Model file for the job. Use its own axes, mm. A direction names the side the tool comes from. Give positions to 0.01 mm unless a question says otherwise; leave off trailing zeros. Order: outer loops, then holes, each group sorted by start corner. A loop starts at its lowest first (then second) coordinate and runs counter-clockwise, first axis right, second up. Notation, with made-up numbers: (83, 27) - (103, 27) arc R24 cw to (103, 56) - close; hole circle Ø9 at (59.25, 47). An arc over 180 degrees is marked (long way). Return JSON: item names as keys, results as strings. Group by question number.
from build123d import *

# Parameters (mm, degrees)
SKETCH1_W           = 25.4
SKETCH1_H           = 25.4
BOSS_EXTRUDE1_DEPTH = 2.54
BOSS_EXTRUDE3_DEPTH = 2.54
SKETCH6_W           = 25.4
SKETCH6_H           = 3.81
CUT_EXTRUDE1_DEPTH  = 51.545361805
SKETCH7_R           = 1
CUT_EXTRUDE2_DEPTH  = 49.742196298


with BuildPart() as part:
    # Sketch1 → Boss-Extrude1 (new body)
    with BuildSketch(Plane.XY):
        with Locations((12.7, -12.7)):
            Rectangle(SKETCH1_W, SKETCH1_H)
    extrude(amount=BOSS_EXTRUDE1_DEPTH)

    # Sketch2 → Boss-Extrude3 (add, symmetric)
    with BuildSketch(Plane(origin=(0, -19.05, 0), x_dir=(1, 0, 0), z_dir=(0, 1, 0))):
        Polygon((2.286, -35.56), (2.286, -2.54), (12.7, -2.54), (23.114, -2.54), (23.114, -35.56), align=None)
    extrude(amount=BOSS_EXTRUDE3_DEPTH, both=True)

    # Sketch6 → Cut-Extrude1 (cut, through all)
    with BuildSketch(Plane.XY.offset(35.56)):
        with Locations((12.7, -23.495)):
            Rectangle(SKETCH6_W, SKETCH6_H)
    extrude(amount=-CUT_EXTRUDE1_DEPTH, mode=Mode.SUBTRACT)

    # Sketch7 → Cut-Extrude2 (cut, through all)
    with BuildSketch(Plane(origin=(0, -21.59, 0), x_dir=(-1, 0, 0), z_dir=(0, -1, 0))):
        with Locations(Location((-12.7, -32.56, 0), (0, 0, 90))):
            Circle(SKETCH7_R)
    extrude(amount=-CUT_EXTRUDE2_DEPTH, mode=Mode.SUBTRACT)


solid = part.part
(1) Slice it at D-D (x = 3). Give the cut face in (y, z).
(2) Drill centre lines: L1, parallel to X at y = -17.65, z = 32.56; L2, parallel to Z at x = 21.25, y = -14.75; L3, parallel to Y at x = 12.25, z = 19.5. Where is each one in solid material? Low to high.
(3) Slice it at C-C (x = 12.7). Give the cut face in (y, z), and give its area (3 significant figures).
(4) Slice it at A-A (z = 32.56). Give the cut face in (x, y).
(5) Drop flat-ended pins along their axis: pin 1 Ø6 at (x, z) = (14.5, 25.5) entering from +Y; pin 2 Ø8 at (x, y) = (8.5, -18) entering from -Z; pin 3 Ø2.5 at (y, z) = (-18, 24.5) entering from +X; pin 4 Ø5.5 at (y, z) = (-19, 17.5) entering from -X. Give the stop position or say it passes through.
(6) Slice it at B-B (y = -18.25). Give the cut face in (x, z), and give its area (3 significant figures).
(7) 3-axis set-ups, long thin cutter, end or side, ignore diameter. For faces 1 (the face through (13, -16.51, 19)), 2 (the face through (23.114, -19, 19)), 3 (the face through (13, -21.59, 18)), 4 (the face through (2.286, -19, 19)): which of +Z, -Z, +X, -X, +Y, -Y reach the whole face in a straight line?
(8) Pull direction Z, two halves, no side cores. Call faces 5 (the face through (13, -19, 35.56)), 6 (the face through (13, 0, 1)), 7 (the face through (13, -19.086, 31.606)): released by +Z, released by -Z, zero draft, split by the parting line, or undercut.
Result set:
{
 "1": {"outline": "(-21.59, 0) - (0, 0) - (0, 2.54) - (-16.51, 2.54) - (-16.51, 35.56) - (-21.59, 35.56) - close"},
 "2": {"L1": "x = 2.29 to 11.7, 13.7 to 23.11", "L2": "z = 0 to 2.54", "L3": "y = -21.59 to -16.51"},
 "3": {"outline": "(-21.59, 0) - (0, 0) - (0, 2.54) - (-16.51, 2.54) - (-16.51, 31.56) - (-21.59, 31.56) - close; (-21.59, 33.56) - (-16.51, 33.56) - (-16.51, 35.56) - (-21.59, 35.56) - close", "area": "212 mm²"},
 "4": {"outline": "(2.29, -21.59) - (11.7, -21.59) - (11.7, -16.51) - (2.29, -16.51) - close; (13.7, -21.59) - (23.11, -21.59) - (23.11, -16.51) - (13.7, -16.51) - close"},
 "5": {"pin 1": "stops at y = -16.51", "pin 2": "stops at z = 0", "pin 3": "stops at x = 23.11", "pin 4": "stops at x = 2.29"},
 "6": {"outline": "(0, 0) - (25.4, 0) - (25.4, 2.54) - (23.11, 2.54) - (23.11, 35.56) - (2.29, 35.56) - (2.29, 2.54) - (0, 2.54) - close; hole circle Ø2 at (12.7, 32.56)", "area": "749 mm²"},
 "7": {"face 1": "+Z, +X, -X, +Y", "face 2": "+Z, +X, +Y, -Y", "face 3": "+Z, -Z, +X, -X, -Y", "face 4": "+Z, -X, +Y, -Y"},
 "8": {"face 5": "released by +Z", "face 6": "zero draft", "face 7": "undercut"}
}
